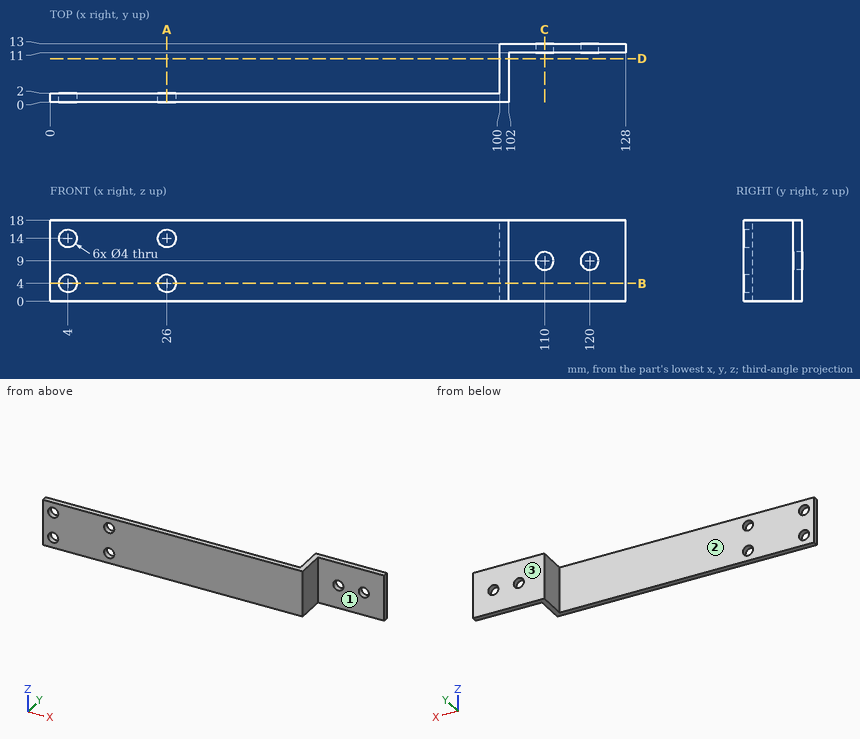
Geometry check sheet. Reference: drawing and pictorial views, mm from the part's lowest x, y, z. A direction names the side the tool comes from. Give positions to 0.01 mm unless a question says otherwise; leave off trailing zeros. Write each loop counter-clockwise with the first axis right and the second up, starting at its lowest first coordinate (ties: lowest second). Pieces come first, ordered by that corner, then holes. Notation, with made-up numbers: M 82.25,41 L 122.25,41 A20 cw 122.25,79 Z; hole C 25.5,33 d8. An arc over 180 degrees is marked long. Put each result on its own line as item: value. Start each with the question number.
1. Section check B-B (z = 4). Record the cut outline in (x, y).
2. Scan lines: line 1 along X through (y, z) = (1.1, 4); line 2 along Z through (x, y) = (4, 1.35); line 3 along Z through (x, y) = (120, 11.8). Record each from-to range of solid material in increasing order. Write a range as [from, to].
3. Section check C-C (x = 110). Record the cut outline in (y, z).
4. Section check A-A (x = 26). Record the cut outline in (y, z), and give its area (3 significant figures).
5. Section check D-D (y = 9.75). Record the cut outline in (x, z).
6. Set-up check for the marked faces 1, 2 and 3: record each of +Z, -Z, +X, -X, +Y, -Y from which the full face is reachable in a straight line by a thin tool's end or side.
7. Go/stop test with flat-tipped pins: pin 1 Ø3 at (y, z) = (8, 12.5) entering from +X; pin 2 Ø9 at (x, z) = (36, 7.5) entering from +Y; pin 3 Ø3.5 at (y, z) = (6.5, 12.5) entering from -X. Record where each tip stops, or that it passes through.
Answer list:
1. outline: M 0,0 L 2,0 L 2,2 L 0,2 Z; M 6,0 L 24,0 L 24,2 L 6,2 Z; M 28,0 L 102,0 L 102,11 L 128,11 L 128,13 L 100,13 L 100,2 L 28,2 Z
2. line 1: [0, 2], [6, 24], [28, 102]
2. line 2: [0, 2], [6, 12], [16, 18]
2. line 3: [0, 7], [11, 18]
3. outline: M 11,0 L 13,0 L 13,7 L 11,7 Z; M 11,11 L 13,11 L 13,18 L 11,18 Z
4. outline: M 0,0 L 2,0 L 2,2 L 0,2 Z; M 0,6 L 2,6 L 2,12 L 0,12 Z; M 0,16 L 2,16 L 2,18 L 0,18 Z
4. area: 20.0 mm2
5. outline: M 100,0 L 102,0 L 102,18 L 100,18 Z
6. face 1: +Z, -Z, +X, -Y
6. face 2: +Z, -Z, -X, +Y
6. face 3: +Z, -Z, +X, -X, +Y
7. pin 1: x = 102
7. pin 2: y = 2
7. pin 3: x = 100
